```python
from build123d import *

# Parameters (mm, degrees)
F1_DEPTH       = 12
F3_D           = 5
F3_CSINK_D     = 10
F3_CSINK_ANGLE = 90
F4_W           = 50
F4_H           = 10
F5_DEPTH       = 25


with BuildPart() as f1:
    # F0 (on Front) → F1 (new body)
    with BuildSketch(Plane.XZ):
        Polygon((0, 110), (0, 0), (375, 0), (375, 46.2607331574), (425, 46.2607331574), (425, 0), (800, 0), (800, 110), align=None)
    extrude(amount=F1_DEPTH)

    # F3 (through all)
    with Locations(Plane.XZ.offset(12)):
        with Locations((35, 6), (185, 6), (615, 6), (765, 6)):
            CounterSinkHole(F3_D / 2, F3_CSINK_D / 2, counter_sink_angle=F3_CSINK_ANGLE)

    # F4 (on face) → F5 (cut)
    with BuildSketch(Plane.XZ.offset(12)):
        with Locations((200, 55)):
            Rectangle(F4_W, F4_H)
        with Locations((600, 55)):
            Rectangle(F4_W, F4_H)
    extrude(amount=-F5_DEPTH, mode=Mode.SUBTRACT)


solid = f1.part
```
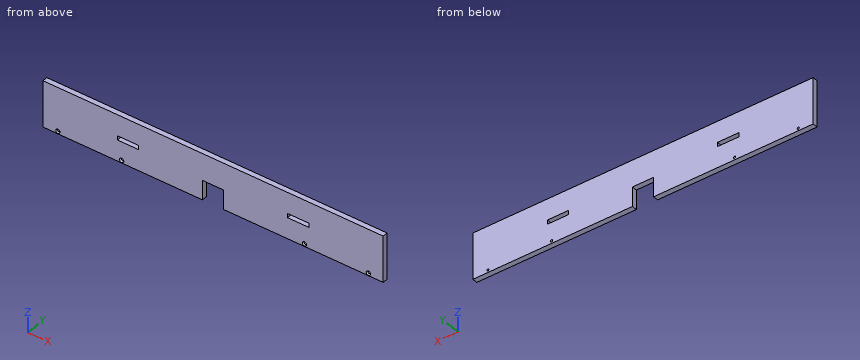
Geometry: final body of the model. Coordinates: model frame, mm. Coordinates: 2 decimals unless noted, no trailing zeros. Order: outer loops, then holes, each group sorted by start corner. A loop starts at its lowest first (then second) coordinate and runs counter-clockwise, first axis right, second up. Notation, with made-up numbers: (63.5, 84.5) -> (76.5, 84.5) arc R13 ccw to (76.5, 103.5) -> close; hole circle Ø5 at (56.25, 21.25). An arc over 180 degrees is marked (long way). Write item = value, one per line.
(1) Line query: line 1 (X direction, y = -9.25, z = 54); line 2 (X direction, y = -6.25, z = 6); line 3 (Z direction, x = 615, y = -4). Output: solid intervals per line, ascending.
Solved:
line_1 = 0 to 175, 225 to 575, 625 to 800
line_2 = 0 to 32.5, 37.5 to 182.5, 187.5 to 375, 425 to 612.5, 617.5 to 762.5, 767.5 to 800
line_3 = 0 to 3.5, 8.5 to 50, 60 to 110
(2) Cut plane A-A on z = 38. Return loops of the section in (x, y).
Solved:
outline = (0, -12) -> (375, -12) -> (375, 0) -> (0, 0) -> close; (425, -12) -> (800, -12) -> (800, 0) -> (425, 0) -> close
(3) Pin query (flat end, axial travel): pin 1 Ø8 at (x, z) = (615, 6) entering from -Y. Return the tip coordinate at first contact, or that it passes through.
Solved:
pin_1 = -11
(4) Cut plane C-C on x = 418. Return loops of the section in (y, z), plus the area to 3 significant figures.
Solved:
outline = (-12, 46.26) -> (0, 46.26) -> (0, 110) -> (-12, 110) -> close
area = 765 mm²
(5) Cut plane B-B on y = -6. Return loops of the section in (x, z), plus the area to 3 significant figures.
Solved:
outline = (0, 0) -> (375, 0) -> (375, 46.26) -> (425, 46.26) -> (425, 0) -> (800, 0) -> (800, 110) -> (0, 110) -> close; hole circle Ø5 at (35, 6); hole (175, 50) -> (225, 50) -> (225, 60) -> (175, 60) -> close; hole circle Ø5 at (185, 6); hole (575, 50) -> (625, 50) -> (625, 60) -> (575, 60) -> close; hole circle Ø5 at (615, 6); hole circle Ø5 at (765, 6)
area = 84,600 mm²
